Check sheet for the modelled part. Datum: model origin and axes. Units: mm. Round coordinates to 2 decimals unless told otherwise and drop trailing zeros. Order: outer loops, then holes, each group sorted by start corner. A loop starts at its lowest first (then second) coordinate and runs counter-clockwise, first axis right, second up. Notation, with made-up numbers: (18, -6.75) -> (75, -6.75) arc R25 cw to (75, 28.25) -> close; hole circle Ø2 at (82.25, 4). An arc over 180 degrees is marked (long way). Answer in a Markdown table with one row per item.
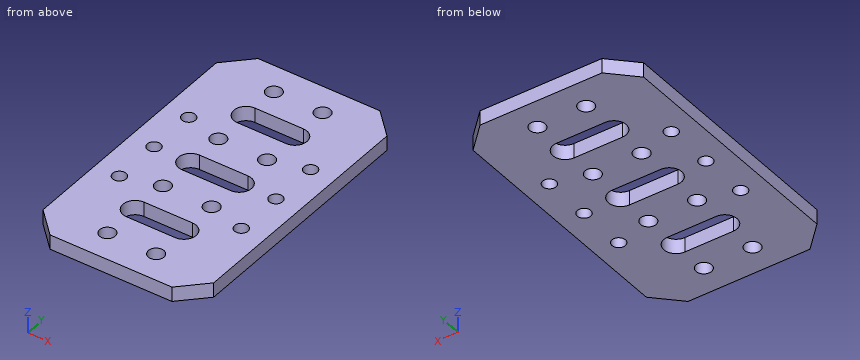
from build123d import *

# Parameters (mm, degrees)
SKETCH_1_W          = 35
SKETCH_1_H          = 60
SKETCH_1_R          = 1.6
EXTRUDE_1_DEPTH     = 3
CUT_EXTRUDE_1_REACH = 5
SKETCH_2_R          = 1.375
CHAMFER_1_SIZE      = 5
CUT_EXTRUDE_2_REACH = 5


with BuildPart() as part:
    # 草图1 → 凸台-拉伸1 (new body)
    with BuildSketch(Plane.XY):
        Rectangle(SKETCH_1_W, SKETCH_1_H)
        with Locations((-5, 8)):
            Circle(SKETCH_1_R, mode=Mode.SUBTRACT)
        with Locations((5, 8)):
            Circle(SKETCH_1_R, mode=Mode.SUBTRACT)
        with Locations((-5, 24)):
            Circle(SKETCH_1_R, mode=Mode.SUBTRACT)
        with Locations((5, 24)):
            Circle(SKETCH_1_R, mode=Mode.SUBTRACT)
        with Locations((-5, -8)):
            Circle(SKETCH_1_R, mode=Mode.SUBTRACT)
        with Locations((5, -8)):
            Circle(SKETCH_1_R, mode=Mode.SUBTRACT)
        with Locations((-5, -24)):
            Circle(SKETCH_1_R, mode=Mode.SUBTRACT)
        with Locations((5, -24)):
            Circle(SKETCH_1_R, mode=Mode.SUBTRACT)
    extrude(amount=EXTRUDE_1_DEPTH)

    # 草图2 → 切除-拉伸1 (cut, up to next)
    with BuildSketch(Plane.XY.offset(3), mode=Mode.PRIVATE) as cut_extrude_1_sk1:
        with Locations((12.5, 0)):
            Circle(SKETCH_2_R)
    cut_extrude_1_tool1 = extrude(cut_extrude_1_sk1.sketch, amount=-CUT_EXTRUDE_1_REACH, mode=Mode.PRIVATE) & part.part
    add(cut_extrude_1_tool1.solids().sort_by_distance((12.5, 0, 3))[0], mode=Mode.SUBTRACT)
    # 草图2 → 切除-拉伸1 (cut, up to next)
    with BuildSketch(Plane.XY.offset(3), mode=Mode.PRIVATE) as cut_extrude_1_sk2:
        with Locations((-12.5, 0)):
            Circle(SKETCH_2_R)
    cut_extrude_1_tool2 = extrude(cut_extrude_1_sk2.sketch, amount=-CUT_EXTRUDE_1_REACH, mode=Mode.PRIVATE) & part.part
    add(cut_extrude_1_tool2.solids().sort_by_distance((-12.5, 0, 3))[0], mode=Mode.SUBTRACT)
    # 草图2 → 切除-拉伸1 (cut, up to next)
    with BuildSketch(Plane.XY.offset(3), mode=Mode.PRIVATE) as cut_extrude_1_sk3:
        with Locations((-12.5, 10)):
            Circle(SKETCH_2_R)
    cut_extrude_1_tool3 = extrude(cut_extrude_1_sk3.sketch, amount=-CUT_EXTRUDE_1_REACH, mode=Mode.PRIVATE) & part.part
    add(cut_extrude_1_tool3.solids().sort_by_distance((-12.5, 10, 3))[0], mode=Mode.SUBTRACT)
    # 草图2 → 切除-拉伸1 (cut, up to next)
    with BuildSketch(Plane.XY.offset(3), mode=Mode.PRIVATE) as cut_extrude_1_sk4:
        with Locations((12.5, 10)):
            Circle(SKETCH_2_R)
    cut_extrude_1_tool4 = extrude(cut_extrude_1_sk4.sketch, amount=-CUT_EXTRUDE_1_REACH, mode=Mode.PRIVATE) & part.part
    add(cut_extrude_1_tool4.solids().sort_by_distance((12.5, 10, 3))[0], mode=Mode.SUBTRACT)
    # 草图2 → 切除-拉伸1 (cut, up to next)
    with BuildSketch(Plane.XY.offset(3), mode=Mode.PRIVATE) as cut_extrude_1_sk5:
        with Locations((-12.5, -10)):
            Circle(SKETCH_2_R)
    cut_extrude_1_tool5 = extrude(cut_extrude_1_sk5.sketch, amount=-CUT_EXTRUDE_1_REACH, mode=Mode.PRIVATE) & part.part
    add(cut_extrude_1_tool5.solids().sort_by_distance((-12.5, -10, 3))[0], mode=Mode.SUBTRACT)
    # 草图2 → 切除-拉伸1 (cut, up to next)
    with BuildSketch(Plane.XY.offset(3), mode=Mode.PRIVATE) as cut_extrude_1_sk6:
        with Locations((12.5, -10)):
            Circle(SKETCH_2_R)
    cut_extrude_1_tool6 = extrude(cut_extrude_1_sk6.sketch, amount=-CUT_EXTRUDE_1_REACH, mode=Mode.PRIVATE) & part.part
    add(cut_extrude_1_tool6.solids().sort_by_distance((12.5, -10, 3))[0], mode=Mode.SUBTRACT)

    # 倒角1
    chamfer_1_edges = [part.edges().sort_by_distance(p)[0] for p in [
        (17.5, -30, 1.5),
        (-17.5, -30, 1.5),
        (-17.5, 30, 1.5),
        (17.5, 30, 1.5),
    ]]
    chamfer(chamfer_1_edges, length=CHAMFER_1_SIZE)

    # 草图3 → 切除-拉伸2 (cut, up to next)
    with BuildSketch(Plane.XY.offset(3), mode=Mode.PRIVATE) as cut_extrude_2_sk1:
        with BuildLine():
            Line((-5, -2.5), (5, -2.5))
            ThreePointArc((5, -2.5), (7.5, 0), (5, 2.5))
            Line((5, 2.5), (-5, 2.5))
            ThreePointArc((-5, 2.5), (-7.5, 0), (-5, -2.5))
        make_face()
    cut_extrude_2_tool1 = extrude(cut_extrude_2_sk1.sketch, amount=-CUT_EXTRUDE_2_REACH, mode=Mode.PRIVATE) & part.part
    add(cut_extrude_2_tool1.solids().sort_by_distance((0, 0, 3))[0], mode=Mode.SUBTRACT)
    # 草图3 → 切除-拉伸2 (cut, up to next)
    with BuildSketch(Plane.XY.offset(3), mode=Mode.PRIVATE) as cut_extrude_2_sk2:
        with BuildLine():
            Line((-5, 13.5), (5, 13.5))
            ThreePointArc((5, 13.5), (7.5, 16), (5, 18.5))
            Line((5, 18.5), (-5, 18.5))
            ThreePointArc((-5, 18.5), (-7.5, 16), (-5, 13.5))
        make_face()
    cut_extrude_2_tool2 = extrude(cut_extrude_2_sk2.sketch, amount=-CUT_EXTRUDE_2_REACH, mode=Mode.PRIVATE) & part.part
    add(cut_extrude_2_tool2.solids().sort_by_distance((0, 16, 3))[0], mode=Mode.SUBTRACT)
    # 草图3 → 切除-拉伸2 (cut, up to next)
    with BuildSketch(Plane.XY.offset(3), mode=Mode.PRIVATE) as cut_extrude_2_sk3:
        with BuildLine():
            Line((-5, -18.5), (5, -18.5))
            ThreePointArc((5, -18.5), (7.5, -16), (5, -13.5))
            Line((5, -13.5), (-5, -13.5))
            ThreePointArc((-5, -13.5), (-7.5, -16), (-5, -18.5))
        make_face()
    cut_extrude_2_tool3 = extrude(cut_extrude_2_sk3.sketch, amount=-CUT_EXTRUDE_2_REACH, mode=Mode.PRIVATE) & part.part
    add(cut_extrude_2_tool3.solids().sort_by_distance((0, -16, 3))[0], mode=Mode.SUBTRACT)


solid = part.part
Item 1: Cross-section at C-C (z = 1.5). State how many separate pieces and enclosed holes the cut face has, and give its area (3 significant figures).
Result sheet:
| item | result |
|---|---|
| separate pieces | 1 |
| enclosed holes | 17 |
| area | 1,740 mm^2 |
Item 2: Cross-section at A-A (y = 0). Record the boundary of the cut face in (x, z) (3 decimals).
Result sheet:
| item | result |
|---|---|
| outline | (-17.5, 0) -> (-13.875, 0) -> (-13.875, 3) -> (-17.5, 3) -> close; (-11.125, 0) -> (-7.5, 0) -> (-7.5, 3) -> (-11.125, 3) -> close; (7.5, 0) -> (11.125, 0) -> (11.125, 3) -> (7.5, 3) -> close; (13.875, 0) -> (17.5, 0) -> (17.5, 3) -> (13.875, 3) -> close |
Item 3: Cross-section at B-B (y = -8). Record the boundary of the cut face in (x, z).
Result sheet:
| item | result |
|---|---|
| outline | (-17.5, 0) -> (-6.6, 0) -> (-6.6, 3) -> (-17.5, 3) -> close; (-3.4, 0) -> (3.4, 0) -> (3.4, 3) -> (-3.4, 3) -> close; (6.6, 0) -> (17.5, 0) -> (17.5, 3) -> (6.6, 3) -> close |
Item 4: Scan lines: line 1 (Y direction, x = 0, z = 0.85); line 2 (Y direction, x = 12.5, z = 1.95) (3 decimals); line 3 (X direction, y = -25, z = 2.45). Record each from-to range of solid material in increasing order. Write a range as [from, to].
Result sheet:
| item | result |
|---|---|
| line 1 | y = [-30, -18.5], [-13.5, -2.5], [2.5, 13.5], [18.5, 30] |
| line 2 | y = [-30, -11.375], [-8.625, -1.375], [1.375, 8.625], [11.375, 30] |
| line 3 | x = [-17.5, -6.25], [-3.75, 3.75], [6.25, 17.5] |
